```python
from build123d import *

# Parameters (mm, degrees)
SKETCH1_R           = 2.286
MAIN_BODY_DEPTH     = 1.5875
SKETCH8_W           = 3.175
SKETCH8_H           = 45
BOSS_EXTRUDE4_DEPTH = 45
BOSS_EXTRUDE5_DEPTH = 3.175
CUT_EXTRUDE2_REACH  = 151.86
SKETCH9_R           = 1.25
CUT_EXTRUDE3_REACH  = 48.587
SKETCH12_R          = 1.5
SKETCH12_R_2        = 1.25


with BuildPart() as part:
    # Sketch1 → Main Body (new body)
    with BuildSketch(Plane(origin=(0, 0, 0), x_dir=(1, 0, 0), z_dir=(0, 1, 0))):
        Polygon((-25.4, 86.995), (-63.43142, 86.995), (-63.43142, 60.96), (-78.74, 60.96), (-78.74, 25.4), (-71.12, 25.4), (-71.12, -25.4), (-78.74, -25.4), (-78.74, -60.96), (-63.43142, -60.96), (-63.43142, -86.995), (-25.4, -86.995), (-25.4, -79.375), (25.4, -79.375), (25.4, -86.995), (63.43142, -86.995), (63.43142, -60.96), (78.74, -60.96), (78.74, -25.4), (71.12, -25.4), (71.12, 25.4), (78.74, 25.4), (78.74, 60.96), (63.43142, 60.96), (63.43142, 86.995), (25.4, 86.995), (25.4, 79.375), (-25.4, 79.375), align=None)
        with Locations((-57.15, 76.2)):
            Circle(SKETCH1_R, mode=Mode.SUBTRACT)
        with Locations((57.15, 76.2)):
            Circle(SKETCH1_R, mode=Mode.SUBTRACT)
        with Locations((57.15, -76.2)):
            Circle(SKETCH1_R, mode=Mode.SUBTRACT)
        with Locations((-57.15, -76.2)):
            Circle(SKETCH1_R, mode=Mode.SUBTRACT)
    extrude(amount=MAIN_BODY_DEPTH)

    # Sketch8 → Boss-Extrude4 (add)
    with BuildSketch(Plane(origin=(0, 1.5875, 0), x_dir=(1, 0, 0), z_dir=(0, 1, 0))):
        with Locations((-69.5325, 0)):
            Rectangle(SKETCH8_W, SKETCH8_H)
    extrude(amount=BOSS_EXTRUDE4_DEPTH)

    # Sketch10 → Boss-Extrude5 (add)
    with BuildSketch(Plane.XY.offset(22.5)):
        Polygon((-67.945, 46.5875), (-67.945, 1.5875), (-55.887286341, 1.5875), align=None)
    boss_extrude5 = extrude(amount=-BOSS_EXTRUDE5_DEPTH)

    # Mirror3: Boss-Extrude5 across plane
    add(boss_extrude5.mirror(Plane.XY))

    # Sketch9 → Cut-Extrude2 (cut, up to next)
    with BuildSketch(Plane.ZY.offset(71.12), mode=Mode.PRIVATE) as cut_extrude2_sk1:
        with BuildLine():
            Line((-19, 35.504854797), (-19, 12.670145203))
            ThreePointArc((-19, 12.670145203), (-17.84383352, 12.048629236), (-16.614967985, 12.510032015))
            Line((-16.614967985, 12.510032015), (-6.160032015, 22.964967985))
            ThreePointArc((-6.160032015, 22.964967985), (-5.69506403, 24.0875), (-6.160032015, 25.210032015))
            Line((-6.160032015, 25.210032015), (-16.614967985, 35.664967985))
            ThreePointArc((-16.614967985, 35.664967985), (-17.84383352, 36.126370764), (-19, 35.504854797))
        make_face()
    cut_extrude2_tool1 = extrude(cut_extrude2_sk1.sketch, amount=-CUT_EXTRUDE2_REACH, mode=Mode.PRIVATE) & part.part
    add(cut_extrude2_tool1.solids().sort_by_distance((-71.12, 24.0875, -14.28057))[0], mode=Mode.SUBTRACT)
    # Sketch9 → Cut-Extrude2 (cut, up to next)
    with BuildSketch(Plane.ZY.offset(71.12), mode=Mode.PRIVATE) as cut_extrude2_sk2:
        with BuildLine():
            ThreePointArc((16.614967985, 12.510032015), (17.84383352, 12.048629236), (19, 12.670145203))
            Line((19, 12.670145203), (19, 35.504854797))
            ThreePointArc((19, 35.504854797), (17.84383352, 36.126370764), (16.614967985, 35.664967985))
            Line((16.614967985, 35.664967985), (6.160032015, 25.210032015))
            ThreePointArc((6.160032015, 25.210032015), (5.69506403, 24.0875), (6.160032015, 22.964967985))
            Line((6.160032015, 22.964967985), (16.614967985, 12.510032015))
        make_face()
    cut_extrude2_tool2 = extrude(cut_extrude2_sk2.sketch, amount=-CUT_EXTRUDE2_REACH, mode=Mode.PRIVATE) & part.part
    add(cut_extrude2_tool2.solids().sort_by_distance((-71.12, 24.0875, 14.28057))[0], mode=Mode.SUBTRACT)
    # Sketch9 → Cut-Extrude2 (cut, up to next)
    with BuildSketch(Plane.ZY.offset(71.12), mode=Mode.PRIVATE) as cut_extrude2_sk3:
        with BuildLine():
            ThreePointArc((-11.577467985, 7.472532015), (-12.038870764, 6.24366648), (-11.417354797, 5.0875))
            Line((-11.417354797, 5.0875), (11.417354797, 5.0875))
            ThreePointArc((11.417354797, 5.0875), (12.038870764, 6.24366648), (11.577467985, 7.472532015))
            Line((11.577467985, 7.472532015), (1.122532015, 17.927467985))
            ThreePointArc((1.122532015, 17.927467985), (0, 18.39243597), (-1.122532015, 17.927467985))
            Line((-1.122532015, 17.927467985), (-11.577467985, 7.472532015))
        make_face()
    cut_extrude2_tool3 = extrude(cut_extrude2_sk3.sketch, amount=-CUT_EXTRUDE2_REACH, mode=Mode.PRIVATE) & part.part
    add(cut_extrude2_tool3.solids().sort_by_distance((-71.12, 9.80693, 0))[0], mode=Mode.SUBTRACT)
    # Sketch9 → Cut-Extrude2 (cut, up to next)
    with BuildSketch(Plane.ZY.offset(71.12), mode=Mode.PRIVATE) as cut_extrude2_sk4:
        with BuildLine():
            Line((11.417354797, 43.0875), (-11.417354797, 43.0875))
            ThreePointArc((-11.417354797, 43.0875), (-12.038870764, 41.93133352), (-11.577467985, 40.702467985))
            Line((-11.577467985, 40.702467985), (-1.122532015, 30.247532015))
            ThreePointArc((-1.122532015, 30.247532015), (0, 29.78256403), (1.122532015, 30.247532015))
            Line((1.122532015, 30.247532015), (11.577467985, 40.702467985))
            ThreePointArc((11.577467985, 40.702467985), (12.038870764, 41.93133352), (11.417354797, 43.0875))
        make_face()
    cut_extrude2_tool4 = extrude(cut_extrude2_sk4.sketch, amount=-CUT_EXTRUDE2_REACH, mode=Mode.PRIVATE) & part.part
    add(cut_extrude2_tool4.solids().sort_by_distance((-71.12, 38.36807, 0))[0], mode=Mode.SUBTRACT)
    # Sketch9 → Cut-Extrude2 (cut, up to next)
    with BuildSketch(Plane.ZY.offset(71.12), mode=Mode.PRIVATE) as cut_extrude2_sk5:
        with Locations((15, 39.087508)):
            Circle(SKETCH9_R)
    cut_extrude2_tool5 = extrude(cut_extrude2_sk5.sketch, amount=-CUT_EXTRUDE2_REACH, mode=Mode.PRIVATE) & part.part
    add(cut_extrude2_tool5.solids().sort_by_distance((-71.12, 39.087508, 15))[0], mode=Mode.SUBTRACT)
    # Sketch9 → Cut-Extrude2 (cut, up to next)
    with BuildSketch(Plane.ZY.offset(71.12), mode=Mode.PRIVATE) as cut_extrude2_sk6:
        with Locations((-15, 39.087508)):
            Circle(SKETCH9_R)
    cut_extrude2_tool6 = extrude(cut_extrude2_sk6.sketch, amount=-CUT_EXTRUDE2_REACH, mode=Mode.PRIVATE) & part.part
    add(cut_extrude2_tool6.solids().sort_by_distance((-71.12, 39.087508, -15))[0], mode=Mode.SUBTRACT)
    # Sketch9 → Cut-Extrude2 (cut, up to next)
    with BuildSketch(Plane.ZY.offset(71.12), mode=Mode.PRIVATE) as cut_extrude2_sk7:
        with Locations((-15, 9.0875)):
            Circle(SKETCH9_R)
    cut_extrude2_tool7 = extrude(cut_extrude2_sk7.sketch, amount=-CUT_EXTRUDE2_REACH, mode=Mode.PRIVATE) & part.part
    add(cut_extrude2_tool7.solids().sort_by_distance((-71.12, 9.0875, -15))[0], mode=Mode.SUBTRACT)
    # Sketch9 → Cut-Extrude2 (cut, up to next)
    with BuildSketch(Plane.ZY.offset(71.12), mode=Mode.PRIVATE) as cut_extrude2_sk8:
        with Locations((15, 9.0875)):
            Circle(SKETCH9_R)
    cut_extrude2_tool8 = extrude(cut_extrude2_sk8.sketch, amount=-CUT_EXTRUDE2_REACH, mode=Mode.PRIVATE) & part.part
    add(cut_extrude2_tool8.solids().sort_by_distance((-71.12, 9.0875, 15))[0], mode=Mode.SUBTRACT)

    # Sketch12 → Cut-Extrude3 (cut, up to next)
    with BuildSketch(Plane.XZ, mode=Mode.PRIVATE) as cut_extrude3_sk1:
        with Locations((-32, -69)):
            Circle(SKETCH12_R)
    cut_extrude3_tool1 = extrude(cut_extrude3_sk1.sketch, amount=-CUT_EXTRUDE3_REACH, mode=Mode.PRIVATE) & part.part
    add(cut_extrude3_tool1.solids().sort_by_distance((-32, 0, -69))[0], mode=Mode.SUBTRACT)
    # Sketch12 → Cut-Extrude3 (cut, up to next)
    with BuildSketch(Plane.XZ, mode=Mode.PRIVATE) as cut_extrude3_sk2:
        with Locations((37, -69)):
            Circle(SKETCH12_R)
    cut_extrude3_tool2 = extrude(cut_extrude3_sk2.sketch, amount=-CUT_EXTRUDE3_REACH, mode=Mode.PRIVATE) & part.part
    add(cut_extrude3_tool2.solids().sort_by_distance((37, 0, -69))[0], mode=Mode.SUBTRACT)
    # Sketch12 → Cut-Extrude3 (cut, up to next)
    with BuildSketch(Plane.XZ, mode=Mode.PRIVATE) as cut_extrude3_sk3:
        with Locations((37, 65)):
            Circle(SKETCH12_R)
    cut_extrude3_tool3 = extrude(cut_extrude3_sk3.sketch, amount=-CUT_EXTRUDE3_REACH, mode=Mode.PRIVATE) & part.part
    add(cut_extrude3_tool3.solids().sort_by_distance((37, 0, 65))[0], mode=Mode.SUBTRACT)
    # Sketch12 → Cut-Extrude3 (cut, up to next)
    with BuildSketch(Plane.XZ, mode=Mode.PRIVATE) as cut_extrude3_sk4:
        with Locations((-32, 65)):
            Circle(SKETCH12_R)
    cut_extrude3_tool4 = extrude(cut_extrude3_sk4.sketch, amount=-CUT_EXTRUDE3_REACH, mode=Mode.PRIVATE) & part.part
    add(cut_extrude3_tool4.solids().sort_by_distance((-32, 0, 65))[0], mode=Mode.SUBTRACT)
    # Sketch12 → Cut-Extrude3 (cut, up to next)
    with BuildSketch(Plane.XZ, mode=Mode.PRIVATE) as cut_extrude3_sk5:
        with Locations((-42.25, 2.75)):
            Circle(SKETCH12_R_2)
    cut_extrude3_tool5 = extrude(cut_extrude3_sk5.sketch, amount=-CUT_EXTRUDE3_REACH, mode=Mode.PRIVATE) & part.part
    add(cut_extrude3_tool5.solids().sort_by_distance((-42.25, 0, 2.75))[0], mode=Mode.SUBTRACT)
    # Sketch12 → Cut-Extrude3 (cut, up to next)
    with BuildSketch(Plane.XZ, mode=Mode.PRIVATE) as cut_extrude3_sk6:
        with Locations((-42.25, 35.25)):
            Circle(SKETCH12_R_2)
    cut_extrude3_tool6 = extrude(cut_extrude3_sk6.sketch, amount=-CUT_EXTRUDE3_REACH, mode=Mode.PRIVATE) & part.part
    add(cut_extrude3_tool6.solids().sort_by_distance((-42.25, 0, 35.25))[0], mode=Mode.SUBTRACT)
    # Sketch12 → Cut-Extrude3 (cut, up to next)
    with BuildSketch(Plane.XZ, mode=Mode.PRIVATE) as cut_extrude3_sk7:
        with Locations((5.25, 2.75)):
            Circle(SKETCH12_R_2)
    cut_extrude3_tool7 = extrude(cut_extrude3_sk7.sketch, amount=-CUT_EXTRUDE3_REACH, mode=Mode.PRIVATE) & part.part
    add(cut_extrude3_tool7.solids().sort_by_distance((5.25, 0, 2.75))[0], mode=Mode.SUBTRACT)
    # Sketch12 → Cut-Extrude3 (cut, up to next)
    with BuildSketch(Plane.XZ, mode=Mode.PRIVATE) as cut_extrude3_sk8:
        with Locations((5.25, 35.25)):
            Circle(SKETCH12_R_2)
    cut_extrude3_tool8 = extrude(cut_extrude3_sk8.sketch, amount=-CUT_EXTRUDE3_REACH, mode=Mode.PRIVATE) & part.part
    add(cut_extrude3_tool8.solids().sort_by_distance((5.25, 0, 35.25))[0], mode=Mode.SUBTRACT)


solid = part.part
```
The listing builds one solid part. Answer for the finished solid, in the listing's coordinates (mm). A direction names the side the tool comes from. Coordinates: 2 decimals unless noted, no trailing zeros. Loops run counter-clockwise (first coordinate to the right, second up) from the corner with the lowest first, then second, coordinate; pieces in that order, holes last. Notation, with made-up numbers: (69.25, 55) - (107.25, 55) arc R16 cw to (107.25, 66) - close; hole circle Ø1 at (37, 85). An arc over 180 degrees is marked (long way). Write item = value, one per line.
1) Determine the mould class of faces 5 (the face through (-61.83, 23.77, 20.93)), 6 (the face through (-69.55, 30.36, -11.31)), 7 (the face through (-59.434, 0.783, -76.301)), 8 (the face through (-1, 0, -1)) for opening direction Y: pulls with the +Y half, pulls with the -Y half, needs draft (parallel to the pull), parting line crosses it, or undercut.
Responses:
face_5 = pulls with the +Y half
face_6 = undercut
face_7 = needs draft
face_8 = pulls with the -Y half
2) Each of these flat-tipped pins is pushed along its axis until it touches: P1, Ø0.8, axis at y = 1, z = 77, coming from the +X side; P2, Ø1.7, axis at y = 1, z = 72, coming from the -X side; P3, Ø1.3, axis at x = -70, y = 0.5, coming from the +Z side; P4, Ø4, axis at x = 57.15, z = -76.2, coming from the -Y side. Where does it stop, or does it pass through?
Responses:
P1 = 63.43
P2 = -63.43
P3 = 60.96
P4 = through
3) Section A-A (z = -76.2) is taken. Determine the outline of the cut face in (x, y).
Responses:
outline = (-63.43, 0) - (-59.44, 0) - (-59.44, 1.59) - (-63.43, 1.59) - close; (-54.86, 0) - (54.86, 0) - (54.86, 1.59) - (-54.86, 1.59) - close; (59.44, 0) - (63.43, 0) - (63.43, 1.59) - (59.44, 1.59) - close
4) Section C-C (x = -5) is taken. Determine the outline of the cut face in (y, z) (1 decimal).
Responses:
outline = (0, -79.4) - (1.6, -79.4) - (1.6, 79.4) - (0, 79.4) - close
5) Section D-D (z = -30.5) is taken. Determine the outline of the cut face in (x, y).
Responses:
outline = (-78.74, 0) - (78.74, 0) - (78.74, 1.59) - (-78.74, 1.59) - close
6) Section B-B (y = 32.5) is taken. Determine the outline of the cut face in (x, z) (3 decimals), plus the area to 3 significant figures.
Responses:
outline = (-71.12, -22.5) - (-64.17, -22.5) - (-64.17, -19.325) - (-67.945, -19.325) - (-67.945, -19) - (-71.12, -19) - close; (-71.12, -13.45) - (-67.945, -13.45) - (-67.945, -3.375) - (-71.12, -3.375) - close; (-71.12, 3.375) - (-67.945, 3.375) - (-67.945, 13.45) - (-71.12, 13.45) - close; (-71.12, 19) - (-67.945, 19) - (-67.945, 19.325) - (-64.17, 19.325) - (-64.17, 22.5) - (-71.12, 22.5) - close
area = 110 mm^2
7) Find the intervals of material crossed by line 1 along X through (y, z) = (1, 65); line 2 along Z through (x, y) = (57.15, 0.35) (3 decimals); line 3 along Z through (x, y) = (-67.5, 26) (3 decimals), in increasing order.
Responses:
line_1 = -63.43 to -33.5, -30.5 to 35.5, 38.5 to 63.43
line_2 = -86.995 to -78.486, -73.914 to 73.914, 78.486 to 86.995
line_3 = -22.5 to -19.325, 19.325 to 22.5
8) Which of the six approach directions +Z, -Z, +X, -X, +Y, -Y give full straight-line access (tool end or side, diameter ignored) to faces 1 (the face through (-69.55, 12.77, -6.28)), 2 (the face through (-65, 19, 22.5)), 3 (the face through (-65, 19, -22.5)), 4 (the face through (-65, 14, -19.325))?
Responses:
face_1 = +X, -X
face_2 = +Z, +X, -X, +Y
face_3 = -Z, +X, -X, +Y
face_4 = +X, +Y
